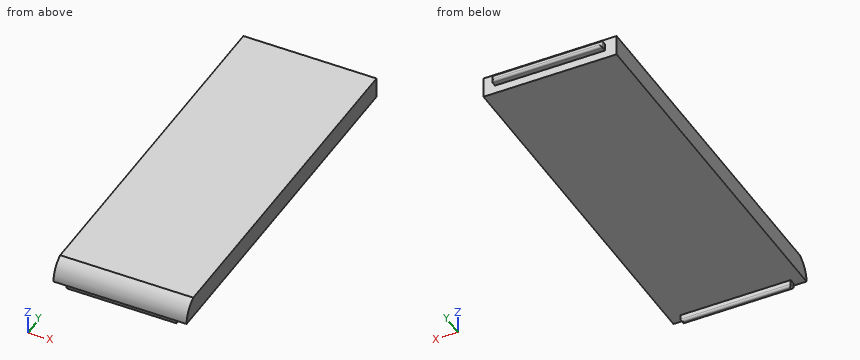
```python
from build123d import *

# Parameters (mm, degrees)
SKETCH1_W           = 57.9
SKETCH1_H           = 160
BOSS_EXTRUDE2_DEPTH = 10
FILLET2_R           = 10
SKETCH2_W           = 47.9
SKETCH2_H           = 2.3
BOSS_EXTRUDE3_DEPTH = 3
FILLET3_R           = 1
SKETCH4_W           = 47.9
SKETCH4_H           = 3
BOSS_EXTRUDE4_DEPTH = 3
FILLET4_R           = 1
SKETCH5_W           = 57.9
SKETCH5_H           = 160
CUT_EXTRUDE1_DEPTH  = 1


with BuildPart() as part:
    # Sketch1 → Boss-Extrude2 (new body)
    with BuildSketch(Plane.XY):
        with Locations((28.95, 80)):
            Rectangle(SKETCH1_W, SKETCH1_H)
    extrude(amount=BOSS_EXTRUDE2_DEPTH)

    # Fillet2
    fillet2_edges = [part.edges().sort_by_distance(p)[0] for p in [
        (28.95, 0, 10),
    ]]
    fillet(fillet2_edges, radius=FILLET2_R - 0.0001)  # a hair under: the kernel refuses the full size

    # Sketch2 → Boss-Extrude3 (add)
    with BuildSketch(Plane(origin=(0, 0, 0), x_dir=(-1, 0, 0), z_dir=(0, 0, -1))):
        with Locations((-28.95, 2.5)):
            Rectangle(SKETCH2_W, SKETCH2_H)
    extrude(amount=BOSS_EXTRUDE3_DEPTH)

    # Fillet3
    fillet3_edges = [part.edges().sort_by_distance(p)[0] for p in [
        (52.9, 2.5, -3),
        (28.95, 1.35, -3),
        (5, 2.5, -3),
        (28.95, 3.65, -3),
    ]]
    fillet(fillet3_edges, radius=FILLET3_R)

    # Sketch4 → Boss-Extrude4 (add)
    with BuildSketch(Plane(origin=(0, 160, 0), x_dir=(1, 0, 0), z_dir=(0, 1, 0))):
        with Locations((28.95, -5.180907412)):
            Rectangle(SKETCH4_W, SKETCH4_H)
    extrude(amount=BOSS_EXTRUDE4_DEPTH)

    # Fillet4
    fillet4_edges = [part.edges().sort_by_distance(p)[0] for p in [
        (5, 163, 5.180907412),
        (28.95, 163, 6.680907412),
        (52.9, 163, 5.180907412),
        (28.95, 163, 3.680907412),
    ]]
    fillet(fillet4_edges, radius=FILLET4_R)

    # Sketch5 → Cut-Extrude1 (cut)
    with BuildSketch(Plane.XY.offset(10)):
        with Locations((28.95, 80)):
            Rectangle(SKETCH5_W, SKETCH5_H)
    extrude(amount=-CUT_EXTRUDE1_DEPTH, mode=Mode.SUBTRACT)


solid = part.part
```
Could you check a few things on this model? Use its own coordinates, in mm. Coordinates: 2 decimals unless noted, no trailing zeros. Loops run counter-clockwise (first coordinate to the right, second up) from the corner with the lowest first, then second, coordinate; pieces in that order, holes last.
1) Imagine slicing it at B-B (y = 101). List the corners of the cut face in (x, z) for me, and give its area (3 significant figures).
Reported:
outline: (0, 0) - (57.9, 0) - (57.9, 9) - (0, 9) - close
area: 521 mm2
2) Imagine slicing it at C-C (z = 2). List the corners of the cut face in (x, y) for me.
Reported:
outline: (0, 0.2) - (57.9, 0.2) - (57.9, 160) - (0, 160) - close
3) Will these pins go through, and if not, where does the flat tip stop? pin 1 Ø1.6 at (y, z) = (3, -1) entering from +X; pin 2 Ø4 at (x, z) = (42, 4.5) entering from -Y; pin 3 Ø2 at (x, z) = (12.5, 2) entering from +Y.
Reported:
pin 1: stops at x = 52.9
pin 2: stops at y = 0.32
pin 3: stops at y = 160
4) Please list where these lines run through material, in increasing order: line 1 along Z through (x, y) = (32.5, 127); line 2 along Y through (x, z) = (34, -1.5); line 3 along Y through (x, z) = (54.5, 8.75).
Reported:
line 1: z = 0 to 9
line 2: y = 1.35 to 3.65
line 3: y = 5.16 to 160
